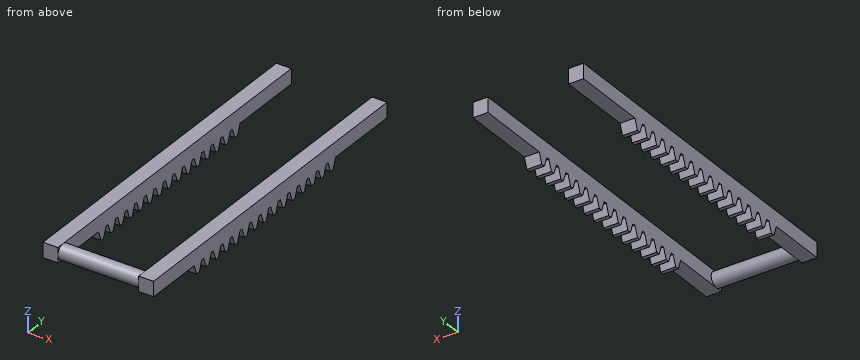
from build123d import *

# Parameters (mm, degrees)
SKETCH_1_W             = 5
SKETCH_1_H             = 5
EXTRUDE_2_DEPTH        = 115
EXTRUDE_2_2_DEPTH      = 115
SKETCH_2_R             = 2.5
EXTRUDE_3_DEPTH        = 27
EXTRUDE_5_DEPTH        = 5
PATTERN_LINEAR_1_COUNT = 15
PATTERN_LINEAR_1_PITCH = 4.71238898
EXTRUDE_6_DEPTH        = 5
PATTERN_LINEAR_2_COUNT = 15
PATTERN_LINEAR_2_PITCH = 4.712


with BuildPart() as part:
    # Sketch 1 → Extrude 2 (new body)
    with BuildSketch(Plane(origin=(0, 0, 0), x_dir=(1, 0, 0), z_dir=(0, 1, 0))):
        with Locations((-18.035714286, 2.5)):
            Rectangle(SKETCH_1_W, SKETCH_1_H)
    extrude(amount=-EXTRUDE_2_DEPTH)



with BuildPart() as body_2:
    # Sketch 1 → Extrude 2 2 (new body)
    with BuildSketch(Plane(origin=(0, 0, 0), x_dir=(1, 0, 0), z_dir=(0, 1, 0))):
        with Locations((13.964285714, 2.5)):
            Rectangle(SKETCH_1_W, SKETCH_1_H)
    extrude(amount=-EXTRUDE_2_2_DEPTH)


with BuildPart() as part_1:
    add(part.part)

    add(body_2.part)  # Extrude 3 merges body 2
    # Sketch 2 → Extrude 3 (add)
    with BuildSketch(Plane(origin=(-15.535714286, 0, 0), x_dir=(0, 0, -1), z_dir=(1, 0, 0))):
        with Locations(Location((2.5, -112.5, 0), (0, 0, 180))):
            Circle(SKETCH_2_R)
    extrude(amount=EXTRUDE_3_DEPTH)

    # Sketch 3 → Extrude 5 (add)
    with BuildSketch(Plane(origin=(16.464285714, 0, 0), x_dir=(0, 0, -1), z_dir=(1, 0, 0))):
        Polygon((5, -91.278917131), (8.375, -92.507316672), (8.375, -93.771600459), (5, -95), align=None)
    extrude_5 = extrude(amount=-EXTRUDE_5_DEPTH)

    # Pattern Linear 1: Extrude 5 ×15
    with Locations(*[(0, i * PATTERN_LINEAR_1_PITCH, 0) for i in range(1, PATTERN_LINEAR_1_COUNT)]):
        add(extrude_5)

    # Sketch 4 → Extrude 6 (add)
    with BuildSketch(Plane.ZY.offset(20.535714286)):
        Polygon((-5, -25.305471406), (-8.375, -26.533870947), (-8.375, -27.798154734), (-5, -29.026554275), align=None)
    extrude_6 = extrude(amount=-EXTRUDE_6_DEPTH)

    # Pattern Linear 2: Extrude 6 ×15
    with Locations(*[(0, -i * PATTERN_LINEAR_2_PITCH, 0) for i in range(1, PATTERN_LINEAR_2_COUNT)]):
        add(extrude_6)


solid = part_1.part
Model file for the job. Use its own axes, mm. Give positions to 0.01 mm unless a question says otherwise; leave off trailing zeros. Order: outer loops, then holes, each group sorted by start corner. A loop starts at its lowest first (then second) coordinate and runs counter-clockwise, first axis right, second up. Notation, with made-up numbers: M 22,0 L 62,0 A13 ccw 62,14 Z; hole C -17,-3 d5. An arc over 180 degrees is marked long. Put each result on its own line as item: value. Start each with the question number.
(1) Band-saw the part on A-A on x = -13. Give the cut face in (y, z).
(2) Pin check, flat tips, straight feed: pin 1 Ø1 at (x, z) = (-12, -7) entering from -Y; pin 2 Ø0.5 at (x, y) = (14, -58) entering from -Z. Stop position of each tip, or through.
(3) Drill centre lines: L1, parallel to X at y = -47, z = -5.5; L2, parallel to Y at x = -9, z = -3.5; L3, parallel to Y at x = 2, z = -3.75. Where is each one in solid material? Low to high. Write a range as [from, to].
Results below:
1. outline: C -112.5,-2.5 d5
2. pin 1: passes through
2. pin 2: stops at z = -5
3. L1: x = [-20.54, -15.54], [11.46, 16.46]
3. L2: y = [-114.79, -110.21]
3. L3: y = [-114.67, -110.33]
